Geometry check sheet. Reference: the model listing, model coordinates, mm. Round coordinates to 2 decimals unless told otherwise and drop trailing zeros. Write each loop counter-clockwise with the first axis right and the second up, starting at its lowest first coordinate (ties: lowest second). Pieces come first, ordered by that corner, then holes. Notation, with made-up numbers: (16.5, 49) -> (37.5, 49) arc R21 ccw to (37.5, 79) -> close; hole circle Ø2 at (12, -30.5). An arc over 180 degrees is marked (long way). Return JSON: item names as keys, results as strings. Group by question number.
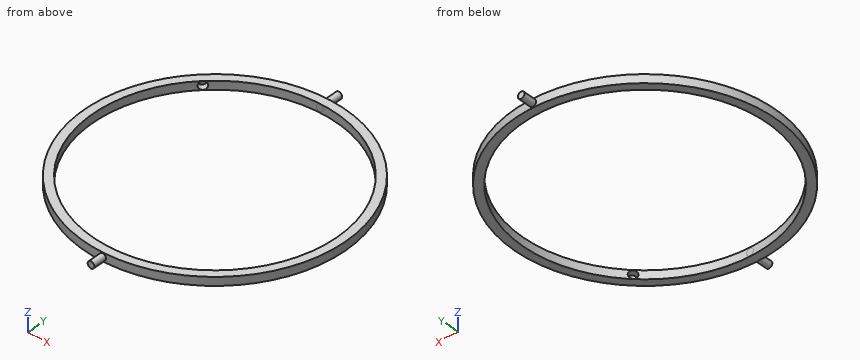
from build123d import *

# Parameters (mm, degrees)
F0_R           = 48.895
F0_R_2         = 45.72
F1_DEPTH       = 3.175
F2_R           = 1.27
F3_DEPTH       = 53.975
F3_DEPTH_BACK  = 53.975
F4_R           = 45.72
F5_DEPTH       = 25.4
F9_R           = 1.524
F10_DEPTH      = 48.26
F10_DEPTH_BACK = 48.26


with BuildPart() as f1:
    # F0 (on Top) → F1 (new body)
    with BuildSketch(Plane.XY):
        Circle(F0_R)
        Circle(F0_R_2, mode=Mode.SUBTRACT)
    extrude(amount=F1_DEPTH)

    # F2 (on Front) → F3 (join, two sides)
    with BuildSketch(Plane.XZ) as f3_sk:
        with Locations((0, 1.5875)):
            Circle(F2_R)
    extrude(amount=F3_DEPTH)
    extrude(f3_sk.sketch, amount=-F3_DEPTH_BACK)

    # F4 (on Top) → F5 (cut)
    with BuildSketch(Plane.XY):
        Circle(F4_R)
    extrude(amount=F5_DEPTH, mode=Mode.SUBTRACT)

    # F9 (on face) → F10 (cut, two sides)
    with BuildSketch(Plane(origin=(0, 0, 0), x_dir=(-0.7071067812, -0.7071067812, 0), z_dir=(-0.7071067812, 0.7071067812, 0))) as f10_sk:
        with Locations((0, 1.5875)):
            Circle(F9_R)
    extrude(amount=-F10_DEPTH, mode=Mode.SUBTRACT)
    extrude(f10_sk.sketch, amount=F10_DEPTH_BACK, mode=Mode.SUBTRACT)


solid = f1.part
1) Material ranges on probe 1 along Y at (x, z) = (0, 2.45) (3 decimals); probe 2 along Y at (x, z) = (10.5, 1.3); probe 3 along X at (y, z) = (40.5, 2.8), recorded low to high. Write a range as [from, to].
2) Sectioned sample at B-B on y = 0. Enter the section's corners in (x, z) (3 decimals).
3) Go/stop test with a flat-tipped pin: P1, Ø1, axis at y = 34, z = 2.5, coming from the +X side. Record where the tip stops, or that it passes through.
4) Sectioned sample at C-C on x = 15. Enter the section's corners in (y, z) (3 decimals).
Evaluation:
{
 "1": {"probe 1": "y = [-53.975, -45.72], [45.72, 53.975]", "probe 2": "y = [-47.75, -44.5], [44.5, 47.75]", "probe 3": "x = [-27.39, -21.21], [21.21, 27.39]"},
 "2": {"outline": "(-48.895, 0) -> (-45.72, 0) -> (-45.72, 3.175) -> (-48.895, 3.175) -> close; (45.72, 0) -> (48.895, 0) -> (48.895, 3.175) -> (45.72, 3.175) -> close"},
 "3": {"P1": "stops at x = 35.62"},
 "4": {"outline": "(-46.537, 0) -> (-43.189, 0) -> (-43.189, 3.175) -> (-46.537, 3.175) -> close; (43.189, 0) -> (46.537, 0) -> (46.537, 3.175) -> (43.189, 3.175) -> close"}
}
